Input: part model. Units: mm. Frame: model coordinates. Face numbers are marked on the shaded views. Coordinates: 2 decimals unless noted, no trailing zeros. Order: outer loops, then holes, each group sorted by start corner. A loop starts at its lowest first (then second) coordinate and runs counter-clockwise, first axis right, second up.
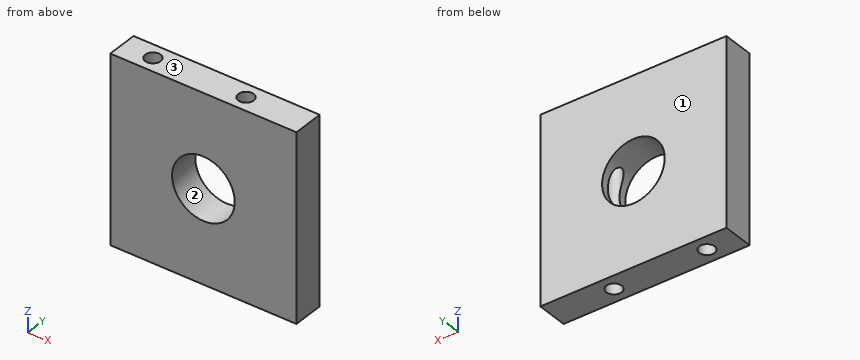
Autodesk Inventor part; units mm, degrees
ref_plane "YZ Plane" through (0, 0, 0) normal (1, 0, 0) x (0, 1, 0)
ref_plane "XZ Plane" through (0, 0, 0) normal (0, 1, 0) x (-1, 0, 0)
ref_plane "XY Plane" through (0, 0, 0) normal (0, 0, 1) x (1, 0, 0)
sketch "スケッチ1" plane through (0, 0, 0) normal (0, 1, 0) x (-1, 0, 0)
  line L0 (0, 0) -> (30, 0)
  line L1 (30, 0) -> (30, -30)
  line L2 (30, -30) -> (0, -30)
  line L3 (0, -30) -> (0, 0)
  dimension "d0" = 30
  dimension "d1" = 30
extrude "押し出し1" add sketch "スケッチ1" along normal blind 5
sketch "スケッチ2" plane through (-30, 0, 0) normal (0, 0, 1) x (1, 0, 0)
  line L0 (0, 0) -> (0, 5)
  line L1 (0, 2.5) -> (30, 2.5)
  line L2 (30, 0) -> (30, 5)
  point P0 (5, 2.5)
  point P1 (20, 2.5)
  dimension "d4" = 10
  dimension "d5" = 15
hole "穴1" at (-25, 2.5, 0) at (-10, 2.5, 0) direction (0, 0, -1) diameter 2.5 end through all
sketch "スケッチ3" plane through (0, 5, 0) normal (0, 1, 0) x (1, 0, 0)
  line L0 (-30, 30) -> (-30, 0)
  line L1 (-30, 15) -> (0, 15)
  line L2 (0, 0) -> (0, 30)
  line L3 (-30, 0) -> (0, 0)
  line L4 (-15, 0) -> (-15, 30)
  line L5 (0, 30) -> (-30, 30)
  circle A0 centre (-15, 15) radius 5.05
  dimension "d13" = 10.1
extrude "押し出し2" cut sketch "スケッチ3" against normal blind 5 contours A0 L4 L1 | L1 L4 A0 | A0 L1 L4 | L1 A0 L4
properties part number "hand2_08" material "アルミニウム 6061-AHC"
Item 1: Cut plane A-A on z = -15. Return loops of the section in (x, y), then the cut area to 3 significant figures.
Response values:
outline: (-30, 0) - (-20.05, 0) - (-20.05, 5) - (-30, 5) - close; (-9.95, 0) - (0, 0) - (0, 5) - (-9.95, 5) - (-9.95, 3.75) arc R1.25 cw to (-9.95, 1.25) - close; hole circle Ø2.5 at (-25, 2.5)
area: 92.3 mm2
Item 2: Draft query along Z for the marked faces 1, 2 and 3. Return one class per face: pulls with the +Z half, pulls with the -Z half, needs draft (parallel to the pull), parting line crosses it, or undercut.
Response values:
face 1: needs draft
face 2: undercut
face 3: pulls with the +Z half
Item 3: Ray query, probe 1 along X at (y, z) = (2.5, -7.5); probe 2 along Y at (x, z) = (-10, -19); probe 3 along X at (y, z) = (1.65, -27). Return the intervals inside material, ascending.
Response values:
probe 1: x = -30 to -26.25, -23.75 to -11.25, -8.75 to 0
probe 2: y = 0 to 1.25, 3.75 to 5
probe 3: x = -30 to -25.92, -24.08 to -10.92, -9.08 to 0
Item 4: Cut plane C-C on y = 2.5. Return loops of the section in (x, z).
Response values:
outline: (-30, -30) - (-26.25, -30) - (-26.25, 0) - (-30, 0) - close; (-23.75, -30) - (-11.25, -30) - (-11.25, -18.38) arc R5.05 cw (long way) to (-11.25, -11.62) - (-11.25, 0) - (-23.75, 0) - close; (-8.75, -30) - (0, -30) - (0, 0) - (-8.75, 0) - close
Item 5: Cut plane B-B on x = -15. Return loops of the section in (y, z), then the cut area to 3 significant figures.
Response values:
outline: (0, -30) - (5, -30) - (5, -20.05) - (0, -20.05) - close; (0, -9.95) - (5, -9.95) - (5, 0) - (0, 0) - close
area: 99.5 mm2
Item 6: Cut plane D-D on z = -18.5. Return loops of the section in (x, y), then the cut area to 3 significant figures.
Response values:
outline: (-30, 0) - (-18.64, 0) - (-18.64, 5) - (-30, 5) - close; (-11.36, 0) - (0, 0) - (0, 5) - (-11.36, 5) - close; hole circle Ø2.5 at (-25, 2.5); hole circle Ø2.5 at (-10, 2.5)
area: 104 mm2
